Geometry check sheet. Reference: drawing and pictorial views, mm from the part's lowest x, y, z. A direction names the side the tool comes from. Give positions to 0.01 mm unless a question says otherwise; leave off trailing zeros. Order: outer loops, then holes, each group sorted by start corner. A loop starts at its lowest first (then second) coordinate and runs counter-clockwise, first axis right, second up.
Item 1: Gauge pin test, flat ends, axial feed: P1, Ø10, axis at x = 58, y = 14.5, coming from the +Z side; P2, Ø3, axis at x = 21, z = 55, coming from the +Y side; P3, Ø16, axis at x = 6.5, y = 12.5, coming from the -Z side. Record the tip position at first contact, or that the pin passes through.
Item 2: Release check for a two-part mould opening along X. For the marked faces 1, 2, 3 and 4 record: released by +X, released by -X, zero draft, split by the parting line, or undercut.
Item 3: Sectioned sample at B-B on y = 18. Record the boundary of the cut face in (x, z), and give its area (3 significant figures).
Item 4: Sectioned sample at D-D on z = 57.5. Record the boundary of the cut face in (x, y).
Item 5: Sectioned sample at A-A on z = 12.5. Record the boundary of the cut face in (x, y), and give its area (3 significant figures).
Item 6: Sectioned sample at C-C on x = 53.75. Record the boundary of the cut face in (y, z).
Item 7: Material ranges on line 1 along X through (y, z) = (1.95, 61.5); line 2 along Y through (x, z) = (10, 39.25); line 3 along X through (y, z) = (20.25, 28), recorded low to high.
Item 8: Access from +Z, -Z, +X, -X, +Y, -Y to the whole of each face (thin tool, end or side, straight path). Record for the marked faces 5, 6 and 7.
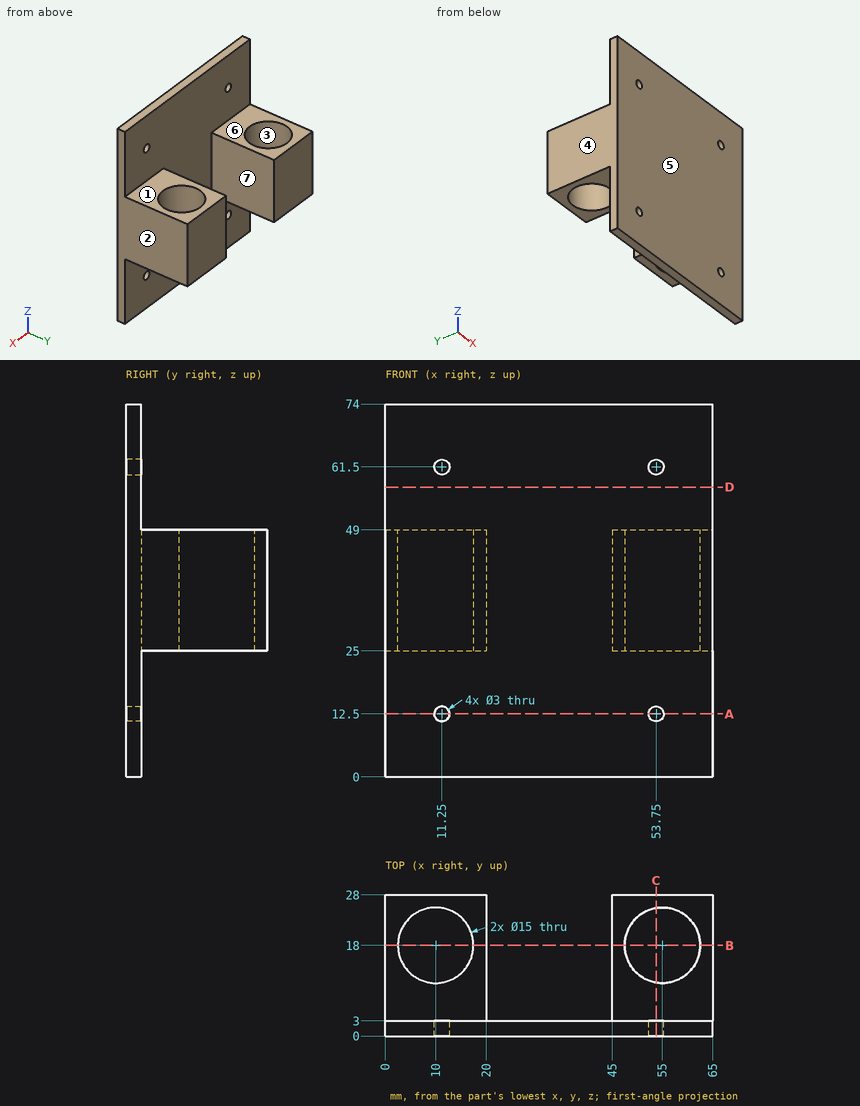
Report:
1. P1: stops at z = 49
1. P2: stops at y = 3
1. P3: stops at z = 25
2. face 1: zero draft
2. face 2: released by +X
2. face 3: undercut
2. face 4: released by -X
3. outline: (0, 25) - (2.5, 25) - (2.5, 49) - (0, 49) - close; (17.5, 25) - (20, 25) - (20, 49) - (17.5, 49) - close; (45, 25) - (47.5, 25) - (47.5, 49) - (45, 49) - close; (62.5, 25) - (65, 25) - (65, 49) - (62.5, 49) - close
3. area: 240 mm2
4. outline: (0, 0) - (65, 0) - (65, 3) - (0, 3) - close
5. outline: (0, 0) - (9.75, 0) - (9.75, 3) - (0, 3) - close; (12.75, 0) - (52.25, 0) - (52.25, 3) - (12.75, 3) - close; (55.25, 0) - (65, 0) - (65, 3) - (55.25, 3) - close
5. area: 177 mm2
6. outline: (0, 0) - (3, 0) - (3, 11) - (0, 11) - close; (0, 14) - (3, 14) - (3, 25) - (10.6, 25) - (10.6, 49) - (3, 49) - (3, 60) - (0, 60) - close; (0, 63) - (3, 63) - (3, 74) - (0, 74) - close; (25.4, 25) - (28, 25) - (28, 49) - (25.4, 49) - close
7. line 1: x = 0 to 9.75, 12.75 to 52.25, 55.25 to 65
7. line 2: y = 0 to 10.5, 25.5 to 28
7. line 3: x = 0 to 2.85, 17.15 to 20, 45 to 47.85, 62.15 to 65
8. face 5: +Z, -Z, +X, -X, -Y
8. face 6: +Z, +X, -X, +Y
8. face 7: +Z, -Z, +Y
